Geometry: final body of the model. Coordinates: model frame, mm. A direction names the side the tool comes from. Round coordinates to 2 decimals unless told otherwise and drop trailing zeros. Loops run counter-clockwise (first coordinate to the right, second up) from the corner with the lowest first, then second, coordinate; pieces in that order, holes last. Notation, with made-up numbers: M -19,89.5 L 8,89.5 A23 ccw 8,120.5 Z; hole C -36,-7 d8. An arc over 180 degrees is marked long. Return JSON: item names as keys, results as strings.
from build123d import *

# Parameters (mm, degrees)
SKETCH_1_W          = 70
SKETCH_1_H          = 80
EXTRUDE_1_DEPTH     = 8
SKETCH_4_R          = 13
CUT_EXTRUDE_2_DEPTH = 8
SKETCH_5_R          = 1.3
CUT_EXTRUDE_3_DEPTH = 10


with BuildPart() as part:
    # 草图1 → 凸台-拉伸1 (new body)
    with BuildSketch(Plane(origin=(0, 0, 0), x_dir=(0, 0, -1), z_dir=(1, 0, 0))):
        Rectangle(SKETCH_1_W, SKETCH_1_H)
    extrude(amount=EXTRUDE_1_DEPTH)

    # 草图4 → 切除-拉伸2 (cut)
    with BuildSketch(Plane(origin=(8, 0, 0), x_dir=(0, 0, -1), z_dir=(1, 0, 0))):
        Circle(SKETCH_4_R)
    extrude(amount=-CUT_EXTRUDE_2_DEPTH, mode=Mode.SUBTRACT)

    # 草图5 → 切除-拉伸3 (cut)
    with BuildSketch(Plane.XY.offset(35)):
        with Locations((4, 34)):
            Circle(SKETCH_5_R)
        with Locations((4, -34.156756408)):
            Circle(SKETCH_5_R)
    cut_extrude_3 = extrude(amount=-CUT_EXTRUDE_3_DEPTH, mode=Mode.SUBTRACT)

    # 镜向1: 切除-拉伸3 across plane
    add(cut_extrude_3.mirror(Plane.XY), mode=Mode.SUBTRACT)


solid = part.part
Q1. Section query B-B (z = 0). Output: boundary loops of the cut face in (x, y).
Determined:
{"outline": "M 0,-40 L 8,-40 L 8,-13 L 0,-13 Z; M 0,13 L 8,13 L 8,40 L 0,40 Z"}
Q2. Section query D-D (y = 34). Output: boundary loops of the cut face in (x, z).
Determined:
{"outline": "M 0,-35 L 2.7,-35 L 2.7,-25 L 5.3,-25 L 5.3,-35 L 8,-35 L 8,35 L 5.3,35 L 5.3,25 L 2.7,25 L 2.7,35 L 0,35 Z"}
Q3. Pull-direction query (X, two-part tool) for faces 4 (the flat face through (4, -1, -35)), 5 (the cylindrical face through (3.83, 35.29, -30.07)), 6 (the flat face through (8, 1, -15)); classes: pulls with the +X half, pulls with the -X half, needs draft (parallel to the pull), parting line crosses it, or undercut.
Determined:
{"face 4": "needs draft", "face 5": "undercut", "face 6": "pulls with the +X half"}
Q4. Section query C-C (x = 4). Output: boundary loops of the cut face in (y, z).
Determined:
{"outline": "M -40,-35 L -35.46,-35 L -35.46,-25 L -32.86,-25 L -32.86,-35 L 32.7,-35 L 32.7,-25 L 35.3,-25 L 35.3,-35 L 40,-35 L 40,35 L 35.3,35 L 35.3,25 L 32.7,25 L 32.7,35 L -32.86,35 L -32.86,25 L -35.46,25 L -35.46,35 L -40,35 Z; hole C 0,0 d26"}
Q5. Pin query (flat end, axial travel): pin 1 (0.8 mm diameter, centred on x = 4, y = 34, fed in from +Z); pin 2 (2.5 mm diameter, centred on x = 4, y = 34, fed in from -Z); pin 3 (2 mm diameter, centred on x = 4, y = -33.5, fed in from -Z). Return the tip coordinate at first contact, or that it passes through.
Determined:
{"pin 1": "stops at z = 25", "pin 2": "stops at z = -25", "pin 3": "stops at z = -35"}
Q6. Material intervals for L1, parallel to Y at x = 4, z = 29; L2, parallel to Y at x = 0.75, z = -0.5; L3, parallel to Y at x = 0.5, z = 12, sorted ascending.
Determined:
{"L1": "y = -40 to -35.46, -32.86 to 32.7, 35.3 to 40", "L2": "y = -40 to -12.99, 12.99 to 40", "L3": "y = -40 to -5, 5 to 40"}
Q7. Reachability of faces 1 (the flat face through (4, -34, -25)), 2 (the cylindrical face through (4.056, -7.91, 10.316)), 3 (the flat face through (4, -34, 25)) from +Z, -Z, +X, -X, +Y, -Y: full face, straight path, thin tool, end or side. Return the list, or none.
Determined:
{"face 1": "-Z", "face 2": "+X, -X", "face 3": "+Z"}
Q8. Section query A-A (y = -5). Output: boundary loops of the cut face in (x, z).
Determined:
{"outline": "M 0,-35 L 8,-35 L 8,-12 L 0,-12 Z; M 0,12 L 8,12 L 8,35 L 0,35 Z"}
